Input: part model. Units: mm. Frame: model coordinates. Coordinates: 2 decimals unless noted, no trailing zeros. Loops run counter-clockwise (first coordinate to the right, second up) from the corner with the lowest first, then second, coordinate; pieces in that order, holes last.
(1) Section A-A, the plane y = 12.25. Return loops of the section in (x, z), then the cut area to 4 significant figures.
(2) Section D-D, the plane y = 6. Return loops of the section in (x, z), then the cut area to 3 significant figures.
(3) Line query: L1, parallel to X at y = 11.5, z = 0.05; L2, parallel to Z at x = 3.5, y = 2.25; L3, parallel to X at y = 10.25, z = -0.6. Output: solid intervals per line, ascending.
(4) Section B-B, the plane x = -2.5. Return loops of the section in (y, z).
(5) Section C-C, the plane z = -0.05. Return loops of the section in (x, y).
```python
from build123d import *

# Parameters (mm, degrees)
SKETCH_1_W          = 7.5
SKETCH_1_H          = 2
EXTRUDE_1_DEPTH     = 13.25
CUT_EXTRUDE_START   = 13.25
SKETCH_2_W          = 0.5
SKETCH_2_H          = 0.5
CUT_EXTRUDE_1_DEPTH = 7
CUT_EXTRUDE_2_DEPTH = 14.806701271


with BuildPart() as part:
    # 草图1 → 凸台-拉伸1 (new body)
    with BuildSketch(Plane(origin=(0, 0, 0), x_dir=(1, 0, 0), z_dir=(0, 1, 0))):
        Rectangle(SKETCH_1_W, SKETCH_1_H)
    extrude(amount=EXTRUDE_1_DEPTH)

    # 草图2 → 切除-拉伸1 (cut)
    with BuildSketch(Plane(origin=(0, 0, 0), x_dir=(1, 0, 0), z_dir=(0, 1, 0)).offset(CUT_EXTRUDE_START)):
        with Locations((2.54, 0)):
            Rectangle(SKETCH_2_W, SKETCH_2_H)
        Rectangle(SKETCH_2_W, SKETCH_2_H)
        with Locations((-2.54, 0)):
            Rectangle(SKETCH_2_W, SKETCH_2_H)
    extrude(amount=-CUT_EXTRUDE_1_DEPTH, mode=Mode.SUBTRACT)

    # 草图3 → 切除-拉伸2 (cut, through all)
    with BuildSketch(Plane(origin=(0, 0, 0), x_dir=(1, 0, 0), z_dir=(0, 1, 0))):
        Polygon((-3.25, -1), (-3.75, -0.5), (-3.75, -1), align=None)
        Polygon((-3.75, 0.5), (-3.25, 1), (-3.75, 1), align=None)
        Polygon((3.75, -0.5), (3.25, -1), (3.75, -1), align=None)
        Polygon((3.25, 1), (3.75, 1), (3.75, 0.5), align=None)
    extrude(amount=CUT_EXTRUDE_2_DEPTH, mode=Mode.SUBTRACT)


solid = part.part
```
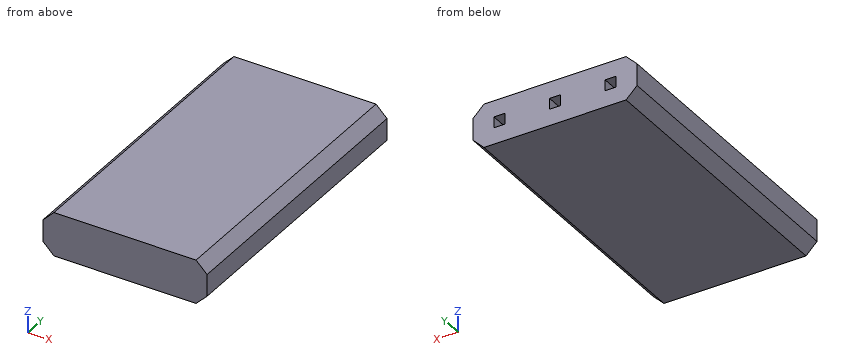
Report:
1. outline: (-3.75, -0.5) - (-3.25, -1) - (3.25, -1) - (3.75, -0.5) - (3.75, 0.5) - (3.25, 1) - (-3.25, 1) - (-3.75, 0.5) - close; hole (-2.79, -0.25) - (-2.29, -0.25) - (-2.29, 0.25) - (-2.79, 0.25) - close; hole (-0.25, -0.25) - (0.25, -0.25) - (0.25, 0.25) - (-0.25, 0.25) - close; hole (2.29, -0.25) - (2.79, -0.25) - (2.79, 0.25) - (2.29, 0.25) - close
1. area: 13.75 mm2
2. outline: (-3.75, -0.5) - (-3.25, -1) - (3.25, -1) - (3.75, -0.5) - (3.75, 0.5) - (3.25, 1) - (-3.25, 1) - (-3.75, 0.5) - close
2. area: 14.5 mm2
3. L1: x = -3.75 to -2.79, -2.29 to -0.25, 0.25 to 2.29, 2.79 to 3.75
3. L2: z = -0.75 to 0.75
3. L3: x = -3.65 to 3.65
4. outline: (0, -1) - (13.25, -1) - (13.25, -0.25) - (6.25, -0.25) - (6.25, 0.25) - (13.25, 0.25) - (13.25, 1) - (0, 1) - close
5. outline: (-3.75, 0) - (3.75, 0) - (3.75, 13.25) - (2.79, 13.25) - (2.79, 6.25) - (2.29, 6.25) - (2.29, 13.25) - (0.25, 13.25) - (0.25, 6.25) - (-0.25, 6.25) - (-0.25, 13.25) - (-2.29, 13.25) - (-2.29, 6.25) - (-2.79, 6.25) - (-2.79, 13.25) - (-3.75, 13.25) - close
